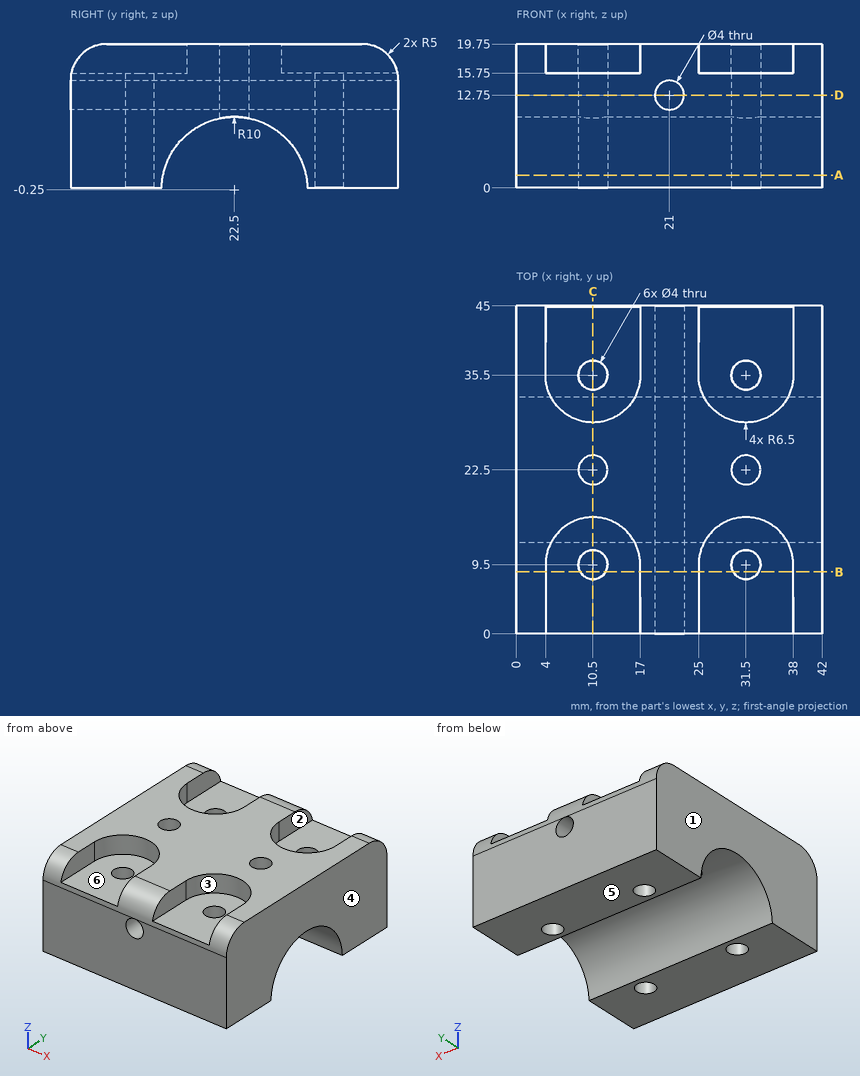
For this review, use the dimensioned drawing (mm, ordinates from the lowest corner) and the shaded views. A direction names the side the tool comes from. Round coordinates to 2 decimals unless told otherwise and drop trailing zeros. Write each loop counter-clockwise with the first axis right and the second up, starting at its lowest first coordinate (ties: lowest second). Pieces come first, ordered by that corner, then holes. Notation, with made-up numbers: (-29.5, -21.75) - (-21.5, -21.75) arc R23 cw to (-21.5, -6.75) - close; hole circle Ø11 at (75, -38.5). An arc over 180 degrees is marked (long way). Answer as a JSON object with one key per item and string values.
1. We need section A-A on z = 1.75. Give the boundary of the cut face in (x, y).
Response values:
{"outline": "(0, 0) - (42, 0) - (42, 12.7) - (0, 12.7) - close; (0, 32.3) - (42, 32.3) - (42, 45) - (0, 45) - close; hole circle Ø4 at (10.5, 9.5); hole circle Ø4 at (10.5, 35.5); hole circle Ø4 at (31.5, 9.5); hole circle Ø4 at (31.5, 35.5)"}
2. Draft analysis for pull direction X (two halves, no side actions). For the marked faces 4, 5 and 6, state which applies: +X half, -X half, draft (parallel to the pull), parting line (faces both ways), or undercut.
Response values:
{"face 4": "+X half", "face 5": "draft", "face 6": "undercut"}
3. Tool access review of the marked faces 1, 2 and 3: name each direction out of +Z, -Z, +X, -X, +Y, -Y from which nothing blocks a thin tool from reaching the whole face with its end or side.
Response values:
{"face 1": "+Z, -Z, -X, +Y, -Y", "face 2": "+Z, +Y", "face 3": "+Z, -Y"}
4. We need section B-B on y = 8.5. Give the boundary of the cut face in (x, z).
Response values:
{"outline": "(0, 0) - (8.77, 0) - (8.77, 15.75) - (4, 15.75) - (4, 19.75) - (0, 19.75) - close; (12.23, 0) - (29.77, 0) - (29.77, 15.75) - (25, 15.75) - (25, 19.75) - (17, 19.75) - (17, 15.75) - (12.23, 15.75) - close; (33.23, 0) - (42, 0) - (42, 19.75) - (38, 19.75) - (38, 15.75) - (33.23, 15.75) - close; hole circle Ø4 at (21, 12.75)"}
5. For pin 1 Ø2 at (x, y) = (5, 29.5) entering from -Z; pin 2 Ø2.5 at (x, y) = (10.5, 9.5) entering from +Z; pin 3 Ø5 at (x, y) = (31.5, 35.5) entering from +Z, all flat-tipped, find the tip position at first contact; note any pin that passes through.
Response values:
{"pin 1": "stops at z = 5.75", "pin 2": "passes through", "pin 3": "stops at z = 15.75"}
6. We need section C-C on x = 10.5. Give the boundary of the cut face in (y, z), then the cut area to 3 significant figures.
Response values:
{"outline": "(0, 0) - (7.5, 0) - (7.5, 15.75) - (0.1, 15.75) arc R5 ccw to (0, 14.75) - close; (11.5, 0) - (12.5, 0) arc R10 cw to (20.5, 9.55) - (20.5, 19.75) - (16, 19.75) - (16, 15.75) - (11.5, 15.75) - close; (24.5, 9.55) arc R10 cw to (32.5, 0) - (33.5, 0) - (33.5, 15.75) - (29, 15.75) - (29, 19.75) - (24.5, 19.75) - close; (37.5, 0) - (45, 0) - (45, 14.75) arc R5 ccw to (44.9, 15.75) - (37.5, 15.75) - close", "area": "442 mm2"}
7. We need section D-D on z = 12.75. Give the boundary of the cut face in (x, y).
Response values:
{"outline": "(0, 0) - (19, 0) - (19, 45) - (0, 45) - close; (23, 0) - (42, 0) - (42, 45) - (23, 45) - close; hole circle Ø4 at (10.5, 9.5); hole circle Ø4 at (10.5, 22.5); hole circle Ø4 at (10.5, 35.5); hole circle Ø4 at (31.5, 9.5); hole circle Ø4 at (31.5, 22.5); hole circle Ø4 at (31.5, 35.5)"}
8. To check wall thickness, follow line 1 along X through (y, z) = (35.5, 10.5); line 2 along X through (y, z) = (17, 12.75); line 3 along X through (y, z) = (8, 10). State the ranges of each line that lie inside material, in increasing order.
Response values:
{"line 1": "x = 0 to 8.5, 12.5 to 29.5, 33.5 to 42", "line 2": "x = 0 to 19, 23 to 42", "line 3": "x = 0 to 9.18, 11.82 to 30.18, 32.82 to 42"}
